Check sheet for the modelled part. Datum: model origin and axes. Units: mm. Face numbers are marked on the shaded views. A direction names the side the tool comes from. Coordinates: 2 decimals unless noted, no trailing zeros. Order: outer loops, then holes, each group sorted by start corner. A loop starts at its lowest first (then second) coordinate and runs counter-clockwise, first axis right, second up. Notation, with made-up numbers: M 48,21 L 56,21 A14 ccw 56,45 Z; hole C 70.25,15.25 d2. An arc over 180 degrees is marked long. Answer in a Markdown table with one row per item. Add a question column.
from build123d import *

# Parameters (mm, degrees)
SKETCH1_W           = 9.525
SKETCH1_H           = 9.525
BOSS_EXTRUDE1_DEPTH = 12.065
SKETCH2_R           = 4.7625
BOSS_EXTRUDE2_DEPTH = 13.335
FILLET1_R           = 0.635
SKETCH3_R           = 5.6515
CUT_EXTRUDE1_DEPTH  = 2.54
SKETCH4_R           = 5.0165
CUT_EXTRUDE2_DEPTH  = 5.588
SKETCH5_R           = 3.81
BOSS_EXTRUDE3_DEPTH = 1.27
FILLET2_R           = 0.635
SKETCH6_R           = 0.889
BOSS_EXTRUDE4_DEPTH = 8.128
FILLET4_R           = 0.381


with BuildPart() as part:
    # Sketch1 → Boss-Extrude1 (new body)
    with BuildSketch(Plane(origin=(0, 0, 0), x_dir=(1, 0, 0), z_dir=(0, 1, 0))):
        Rectangle(SKETCH1_W, SKETCH1_H)
    extrude(amount=-BOSS_EXTRUDE1_DEPTH)

    # Sketch2 → Boss-Extrude2 (add)
    with BuildSketch(Plane(origin=(0, 0, 0), x_dir=(1, 0, 0), z_dir=(0, 1, 0))):
        Circle(SKETCH2_R)
    extrude(amount=BOSS_EXTRUDE2_DEPTH)

    # Fillet1
    fillet1_edges = [part.edges().sort_by_distance(p)[0] for p in [
        (-4.7625, 13.335, 0),
    ]]
    fillet(fillet1_edges, radius=FILLET1_R)

    # Sketch3 → Cut-Extrude1 (cut)
    with BuildSketch(Plane.XZ.offset(12.065)):
        Circle(SKETCH3_R)
    extrude(amount=-CUT_EXTRUDE1_DEPTH, mode=Mode.SUBTRACT)

    # Sketch4 → Cut-Extrude2 (cut)
    with BuildSketch(Plane.XZ.offset(9.525)):
        Circle(SKETCH4_R)
    extrude(amount=-CUT_EXTRUDE2_DEPTH, mode=Mode.SUBTRACT)

    # Sketch5 → Boss-Extrude3 (add)
    with BuildSketch(Plane.XZ.offset(3.937)):
        Circle(SKETCH5_R)
    extrude(amount=BOSS_EXTRUDE3_DEPTH)

    # Fillet2
    fillet2_edges = [part.edges().sort_by_distance(p)[0] for p in [
        (-3.81, -5.207, 0),
    ]]
    fillet(fillet2_edges, radius=FILLET2_R)

    # Sketch6 → Boss-Extrude4 (add)
    with BuildSketch(Plane.XZ.offset(3.937)):
        Circle(SKETCH6_R)
    extrude(amount=BOSS_EXTRUDE4_DEPTH)

    # Fillet4
    fillet4_edges = [part.edges().sort_by_distance(p)[0] for p in [
        (4.7625, -6.0325, 4.7625),
        (-4.7625, -6.0325, 4.7625),
        (-4.7625, -6.0325, -4.7625),
        (4.7625, -6.0325, -4.7625),
    ]]
    fillet(fillet4_edges, radius=FILLET4_R)


solid = part.part
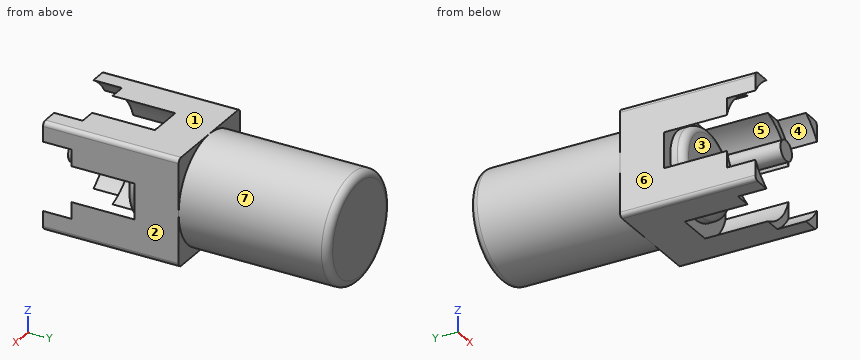
1. Section check A-A on y = -6.5. Enter the section's corners in (x, z), then the cut area to 3 significant figures.
2. Release check for a two-part mould opening along Z. For the marked faces 1, 2, 3 and 4 record: released by +Z, released by -Z, zero draft, split by the parting line, or undercut.
3. Section check B-B on y = 5.25. Enter the section's corners in (x, z) (1 decimal).
4. Scan lines: line 1 (Y direction, x = 0, z = 1.5) (3 decimals); line 2 (Z direction, x = 3, y = -6); line 3 (X direction, y = -6.25, z = 2). Record each from-to range of solid material in increasing order.
5. Go/stop test with flat-tipped pins: pin 1 Ø1.6 at (x, z) = (-3, -3.5) entering from -Y (3 decimals); pin 2 Ø2.5 at (x, z) = (4, -3.5) entering from -Y (3 decimals). Record where each tip stops, or that it passes through.
6. Set-up check for the marked faces 5, 6 and 7: record each of +Z, -Z, +X, -X, +Y, -Y from which the full face is reachable in a straight line by a thin tool's end or side.
Result sheet:
| question | item | result |
|---|---|---|
| 1 | outline | M -4.76,-4.38 A0.38 ccw -4.38,-4.76 L -1.58,-4.76 A5.02 cw -4.76,-1.58 Z; M -4.76,1.58 A5.02 cw -1.58,4.76 L -4.38,4.76 A0.38 ccw -4.76,4.38 Z; C 0,0 d1.78; M 1.58,-4.76 L 4.38,-4.76 A0.38 ccw 4.76,-4.38 L 4.76,-1.58 A5.02 cw Z; M 1.58,4.76 A5.02 cw 4.76,1.58 L 4.76,4.38 A0.38 ccw 4.38,4.76 Z |
| 1 | area | 16.2 mm^2 |
| 2 | face 1 | released by +Z |
| 2 | face 2 | zero draft |
| 2 | face 3 | undercut |
| 2 | face 4 | undercut |
| 3 | outline | C 0,0 d9.5 |
| 4 | line 1 | -5.207 to 13.335 |
| 4 | line 2 | -4.76 to -4.02, 4.02 to 4.76 |
| 4 | line 3 | -4.76 to -4.6, 4.6 to 4.76 |
| 5 | pin 1 | y = -9.525 |
| 5 | pin 2 | y = -12.065 |
| 6 | face 5 | -Y |
| 6 | face 6 | +Z, -Z, -X, +Y, -Y |
| 6 | face 7 | +Y |
